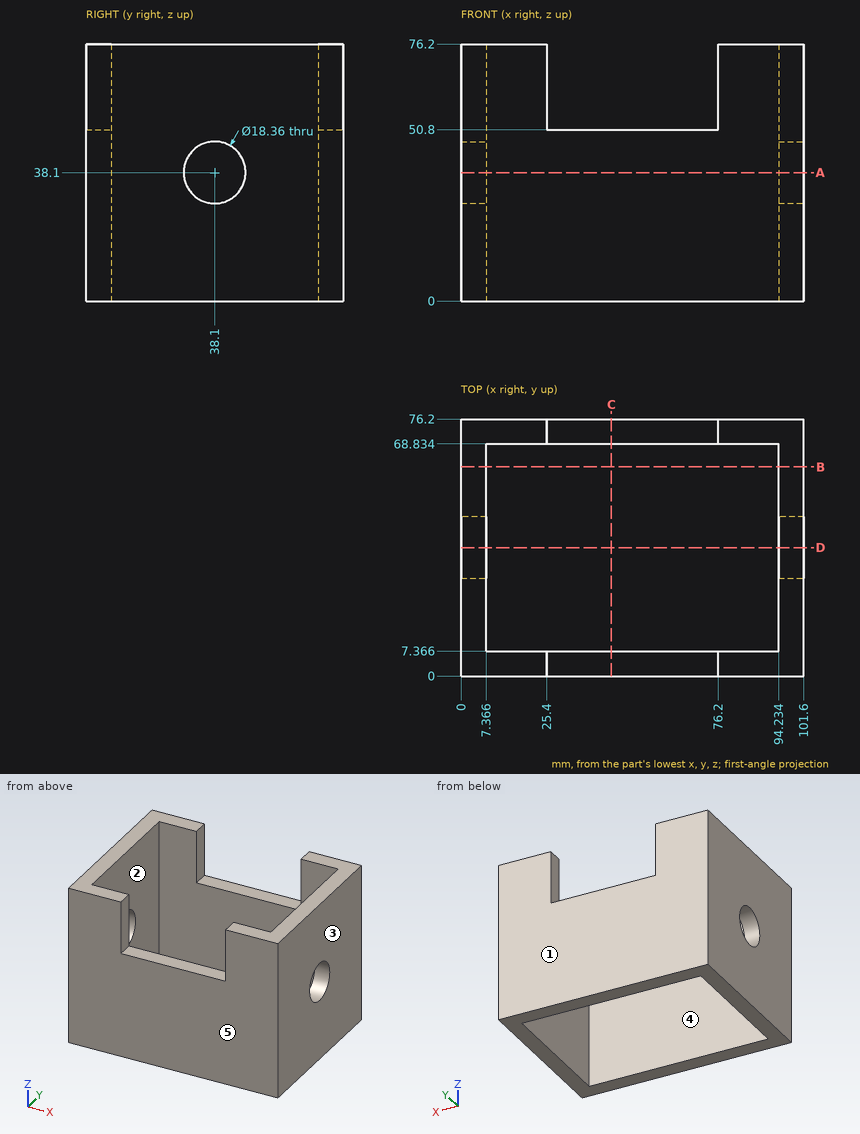
Geometry: see drawing. Coordinates: mm, zero at the bounding-box minimum. A direction names the side the tool comes from. Coordinates: 2 decimals unless noted, no trailing zeros. Loops run counter-clockwise (first coordinate to the right, second up) from the corner with the lowest first, then second, coordinate; pieces in that order, holes last. Notation, with made-up numbers: M -5,-33.5 L 36,-33.5 A9 cw 36,-25.5 Z; hole C 42,16.5 d11. An arc over 180 degrees is marked long. Answer in a Markdown table with one row per item.
1. Section C-C, the plane x = 44.5. Output: boundary loops of the cut face in (y, z).
Response:
| item | result |
|---|---|
| outline | M 0,0 L 7.37,0 L 7.37,50.8 L 0,50.8 Z; M 68.83,0 L 76.2,0 L 76.2,50.8 L 68.83,50.8 Z |
2. Draft query along X for the marked faces 1, 2 and 3. Return one class per face: pulls with the +X half, pulls with the -X half, needs draft (parallel to the pull), parting line crosses it, or undercut.
Response:
| item | result |
|---|---|
| face 1 | needs draft |
| face 2 | undercut |
| face 3 | pulls with the +X half |
3. Material intervals for line 1 (X direction, y = 32.5, z = 64); line 2 (X direction, y = 3.5, z = 73); line 3 (Y direction, x = 78.5, z = 56), sorted ascending.
Response:
| item | result |
|---|---|
| line 1 | x = 0 to 7.37, 94.23 to 101.6 |
| line 2 | x = 0 to 25.4, 76.2 to 101.6 |
| line 3 | y = 0 to 7.37, 68.83 to 76.2 |
4. Reachability of the marked faces 4 and 5 from +Z, -Z, +X, -X, +Y, -Y: full face, straight path, thin tool, end or side. Return the list, or none.
Response:
| item | result |
|---|---|
| face 4 | +Z, -Z |
| face 5 | +Z, -Z, +X, -X, -Y |
5. Section D-D, the plane y = 38.1. Output: boundary loops of the cut face in (x, z).
Response:
| item | result |
|---|---|
| outline | M 0,0 L 7.37,0 L 7.37,28.92 L 0,28.92 Z; M 0,47.28 L 7.37,47.28 L 7.37,76.2 L 0,76.2 Z; M 94.23,0 L 101.6,0 L 101.6,28.92 L 94.23,28.92 Z; M 94.23,47.28 L 101.6,47.28 L 101.6,76.2 L 94.23,76.2 Z |
6. Section A-A, the plane z = 38.1. Output: boundary loops of the cut face in (x, y), then the cut area to 3 significant figures.
Response:
| item | result |
|---|---|
| outline | M 0,0 L 101.6,0 L 101.6,28.92 L 94.23,28.92 L 94.23,7.37 L 7.37,7.37 L 7.37,28.92 L 0,28.92 Z; M 0,47.28 L 7.37,47.28 L 7.37,68.83 L 94.23,68.83 L 94.23,47.28 L 101.6,47.28 L 101.6,76.2 L 0,76.2 Z |
| area | 2,130 mm2 |
7. Section B-B, the plane y = 62. Output: boundary loops of the cut face in (x, z).
Response:
| item | result |
|---|---|
| outline | M 0,0 L 7.37,0 L 7.37,76.2 L 0,76.2 Z; M 94.23,0 L 101.6,0 L 101.6,76.2 L 94.23,76.2 Z |
8. First-contact query: pin 1 (16.5 mm diameter, centred on y = 38.1, z = 38.1, fed in from +X); pin 2 (8 mm diameter, centred on x = 57.5, y = 73, fed in from +Z). Flat tips, straight axial feed; report the tip coordinate or a pass-through.
Response:
| item | result |
|---|---|
| pin 1 | passes through |
| pin 2 | stops at z = 50.8 |
